Check sheet for the drawn part. Datum: minimum x, y, z corner. Units: mm. A direction names the side the tool comes from. Give positions to 0.01 mm unless a question says otherwise; leave off trailing zeros. Write each loop counter-clockwise with the first axis right and the second up, starting at its lowest first coordinate (ties: lowest second). Pieces come first, ordered by that corner, then holes. Notation, with made-up numbers: (68, 51) - (89, 51) arc R26 ccw to (89, 83) - close; hole circle Ø2 at (75, 71.25). An arc over 180 degrees is marked (long way). Use a Markdown table: item, result.
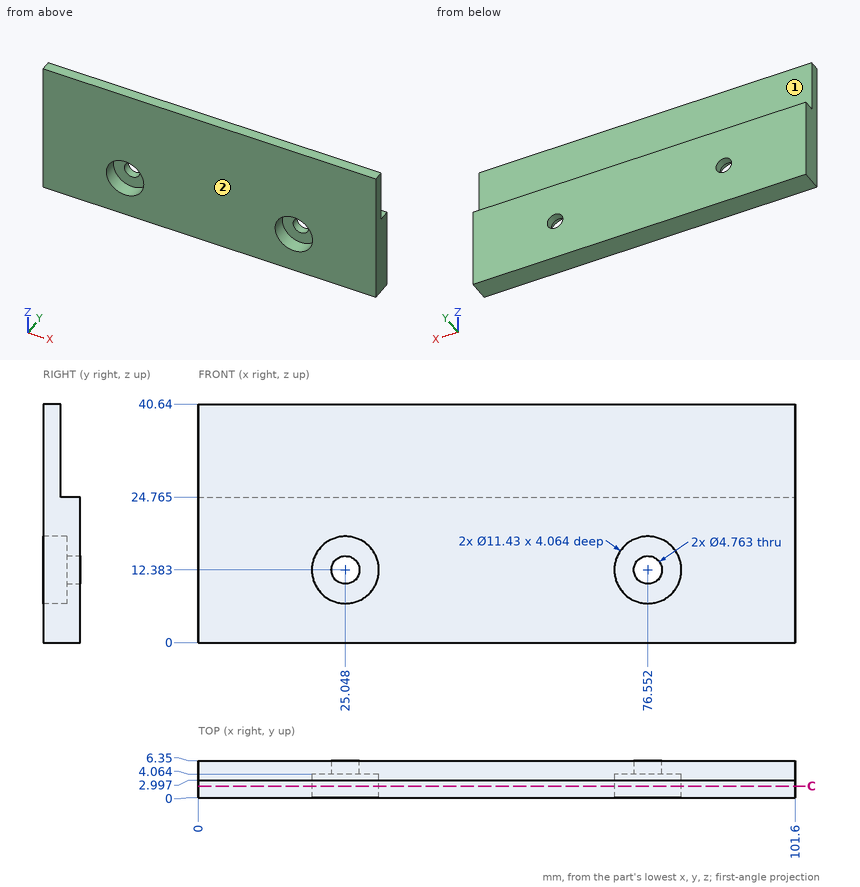
1) Set-up check for the marked faces 1 and 2: record each of +Z, -Z, +X, -X, +Y, -Y from which the full face is reachable in a straight line by a thin tool's end or side.
Working result:
| item | result |
|---|---|
| face 1 | +Z, +X, -X, +Y |
| face 2 | +Z, -Z, +X, -X, -Y |
2) Depth check by flat-ended pin: P1, Ø5.5, axis at x = 76, z = 10, coming from the -Y side; P2, Ø2.5, axis at x = 28.5, y = 4.5, coming from the +Z side (1 decimal). Enter the tip coordinate at first touch or a pass-through.
Working result:
| item | result |
|---|---|
| P1 | stops at y = 4.06 |
| P2 | stops at z = 24.8 |
3) Material ranges on L1, parallel to X at y = 0.75, z = 17.5 (1 decimal); L2, parallel to X at y = 1, z = 13.5; L3, parallel to Z at x = 56, y = 4.25 (1 decimal), recorded low to high. Write a range as from..to.
Working result:
| item | result |
|---|---|
| L1 | x = 0..22.5, 27.6..74, 79.1..101.6 |
| L2 | x = 0..19.44, 30.65..70.95, 82.16..101.6 |
| L3 | z = 0..24.8 |
4) Section check C-C on y = 2. Record the boundary of the cut face in (x, z) (1 decimal).
Working result:
| item | result |
|---|---|
| outline | (0, 0) - (101.6, 0) - (101.6, 40.6) - (0, 40.6) - close; hole circle Ø11.4 at (25, 12.4); hole circle Ø11.4 at (76.6, 12.4) |
